```python
from build123d import *

# Parameters (mm, degrees)
SKETCH1_W            = 76
SKETCH1_H            = 115
BOSS_EXTRUDE1_DEPTH  = 4
M5_CLEARANCE_HOLE1_D = 5.3
FILLET1_R            = 5


with BuildPart() as part:
    # Sketch1 → Boss-Extrude1 (new body)
    with BuildSketch(Plane.XY):
        with Locations((0, 27.5)):
            Rectangle(SKETCH1_W, SKETCH1_H)
    extrude(amount=BOSS_EXTRUDE1_DEPTH)

    # M5 Clearance Hole1 (through all)
    with Locations(Plane.XY.offset(4)):
        with Locations((-23, 67.5), (-23, -15), (23, -15), (23, 67.5)):
            Hole(M5_CLEARANCE_HOLE1_D / 2)

    # Fillet1
    fillet1_edges = [part.edges().sort_by_distance(p)[0] for p in [
        (-38, 85, 2),
        (38, 85, 2),
        (38, -30, 2),
        (-38, -30, 2),
    ]]
    fillet(fillet1_edges, radius=FILLET1_R)


solid = part.part
```
Model file for the job. Use its own axes, mm. Coordinates: 2 decimals unless noted, no trailing zeros. Loops run counter-clockwise (first coordinate to the right, second up) from the corner with the lowest first, then second, coordinate; pieces in that order, holes last. Notation, with made-up numbers: (-26.75, -0.75) -> (28.25, -0.75) arc R10 cw to (28.25, 18.25) -> close; hole circle Ø10 at (-12.75, -28.75). An arc over 180 degrees is marked (long way). Answer as a JSON object with one key per item and string values.
Q1. Flat gauge pin, fed straight in: P1, Ø4, axis at x = -23, y = -15, coming from the -Z side. Where does the tip first touch, or does it go through?
Report:
{"P1": "passes through"}
Q2. Cut at B-B (y = 67.5). List the corners of the cut face in (x, z), and give its area (3 significant figures).
Report:
{"outline": "(-38, 0) -> (-25.65, 0) -> (-25.65, 4) -> (-38, 4) -> close; (-20.35, 0) -> (20.35, 0) -> (20.35, 4) -> (-20.35, 4) -> close; (25.65, 0) -> (38, 0) -> (38, 4) -> (25.65, 4) -> close", "area": "262 mm2"}
Q3. Probe probe 1 along Y at (x, z) = (-23, 1); probe 2 along X at (y, z) = (69, 1.6); probe 3 along Y at (x, z) = (-22, 0.6). List the from-to ranges inside material, lowest first.
Report:
{"probe 1": "y = -30 to -17.65, -12.35 to 64.85, 70.15 to 85", "probe 2": "x = -38 to -25.18, -20.82 to 20.82, 25.18 to 38", "probe 3": "y = -30 to -17.45, -12.55 to 65.05, 69.95 to 85"}
Q4. Pull direction Y, two halves, no side cores. Call faces 1 (the cylindrical face through (36, 84, 2)), 2 (the cylindrical face through (21.777, -17.351, 1.972)), 3 (the flat face through (-38, 27, 2)): released by +Y, released by -Y, zero draft, split by the parting line, or undercut.
Report:
{"face 1": "released by +Y", "face 2": "undercut", "face 3": "zero draft"}
Q5. Cut at A-A (x = -23). List the corners of the cut face in (y, z).
Report:
{"outline": "(-30, 0) -> (-17.65, 0) -> (-17.65, 4) -> (-30, 4) -> close; (-12.35, 0) -> (64.85, 0) -> (64.85, 4) -> (-12.35, 4) -> close; (70.15, 0) -> (85, 0) -> (85, 4) -> (70.15, 4) -> close"}
